Answer from the drawing. Dimensions are ordinates in mm from the lowest x, y and z of the part. A direction names the side the tool comes from. Coordinates: 2 decimals unless noted, no trailing zeros. Order: outer loops, then holes, each group sorted by start corner. A loop starts at its lowest first (then second) coordinate and runs counter-clockwise, first axis right, second up. Notation, with made-up numbers: M 68,-19.75 L 109,-19.75 A23 cw 109,16.25 Z; hole C -26,-22 d1. An arc over 180 degrees is marked long. Use a Markdown table: item, result.
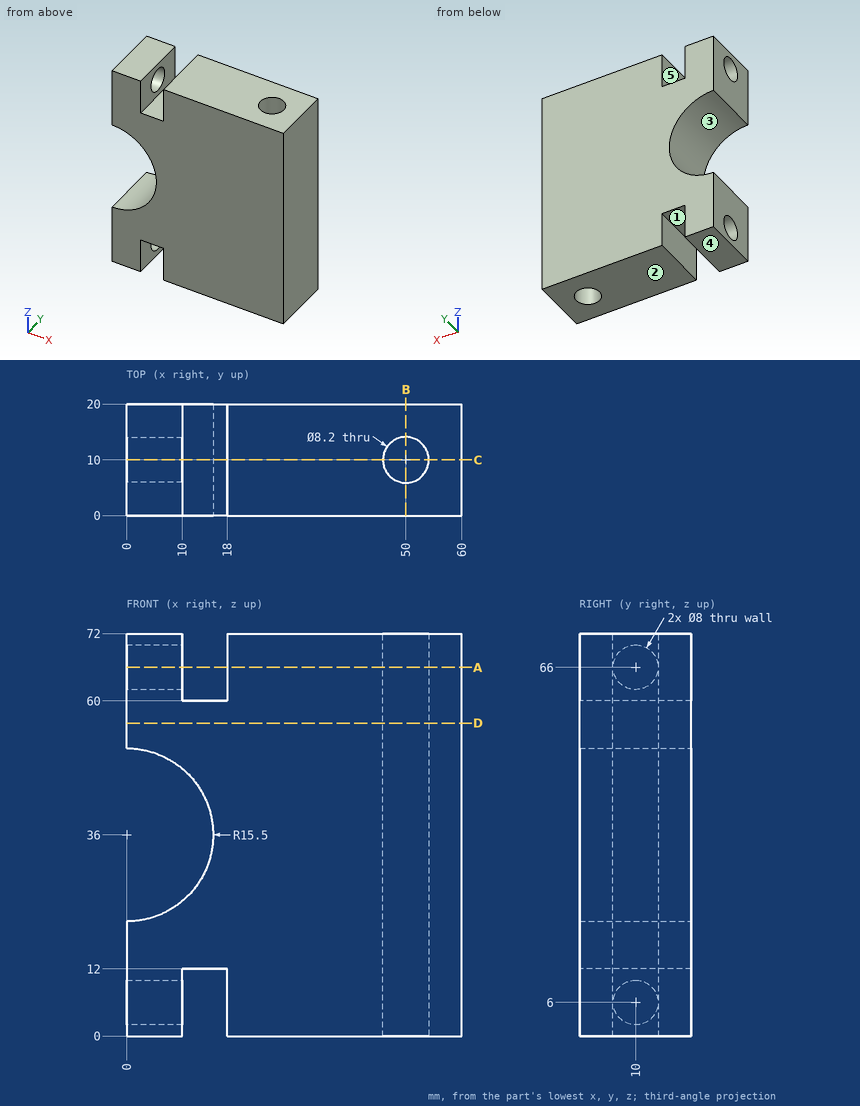
(1) A cutting plane is placed at B-B (x = 50). Determine the outline of the cut face in (y, z).
Conclusion:
| item | result |
|---|---|
| outline | M 0,0 L 5.9,0 L 5.9,72 L 0,72 Z; M 14.1,0 L 20,0 L 20,72 L 14.1,72 Z |
(2) A cutting plane is placed at A-A (z = 66). Determine the outline of the cut face in (x, y).
Conclusion:
| item | result |
|---|---|
| outline | M 0,0 L 10,0 L 10,6 L 0,6 Z; M 0,14 L 10,14 L 10,20 L 0,20 Z; M 18,0 L 60,0 L 60,20 L 18,20 Z; hole C 50,10 d8.2 |
(3) Determine the mould class of the marked faces 3, 4 and 5 for opening direction X: pulls with the +X half, pulls with the -X half, needs draft (parallel to the pull), parting line crosses it, or undercut.
Conclusion:
| item | result |
|---|---|
| face 3 | pulls with the -X half |
| face 4 | needs draft |
| face 5 | undercut |
(4) Given P1, Ø8, axis at x = 21.5, y = 10, coming from the -Z side; P2, Ø2.5, axis at x = 14, y = 8, coming from the +Z side; P3, Ø8, axis at y = 13, z = 36, coming from the -X side (3 decimals); P4, Ø2.5, axis at x = 16, y = 14.5, coming from the -Z side, each flat-ended and moving along its own axis, determine where each tip first touches the part or whether it passes through.
Conclusion:
| item | result |
|---|---|
| P1 | z = 0 |
| P2 | z = 60 |
| P3 | x = 14.975 |
| P4 | z = 12 |
(5) Straight lines are drawn through the part: L1, parallel to Y at x = 4.25, z = 6; L2, parallel to X at y = 9.75, z = 8; L3, parallel to Y at x = 50, z = 24.5. For each, find the intervals that lie inside material, in ascending order.
Conclusion:
| item | result |
|---|---|
| L1 | 0 to 6, 14 to 20 |
| L2 | 18 to 45.91, 54.09 to 60 |
| L3 | 0 to 5.9, 14.1 to 20 |
(6) Which of the six approach directions +Z, -Z, +X, -X, +Y, -Y give full straight-line access (tool end or side, diameter ignored) to the marked faces 1 and 2?
Conclusion:
| item | result |
|---|---|
| face 1 | -Z, +Y, -Y |
| face 2 | -Z, +X, -X, +Y, -Y |
(7) A cutting plane is placed at D-D (z = 56). Determine the outline of the cut face in (x, y), then the cut area to 3 significant figures.
Conclusion:
| item | result |
|---|---|
| outline | M 0,0 L 60,0 L 60,20 L 0,20 Z; hole C 50,10 d8.2 |
| area | 1,150 mm2 |
(8) A cutting plane is placed at C-C (y = 10). Determine the outline of the cut face in (x, z).
Conclusion:
| item | result |
|---|---|
| outline | M 0,0 L 10,0 L 10,2 L 0,2 Z; M 0,10 L 10,10 L 10,12 L 18,12 L 18,0 L 45.9,0 L 45.9,72 L 18,72 L 18,60 L 10,60 L 10,62 L 0,62 L 0,51.5 A15.5 cw 0,20.5 Z; M 0,70 L 10,70 L 10,72 L 0,72 Z; M 54.1,0 L 60,0 L 60,72 L 54.1,72 Z |
